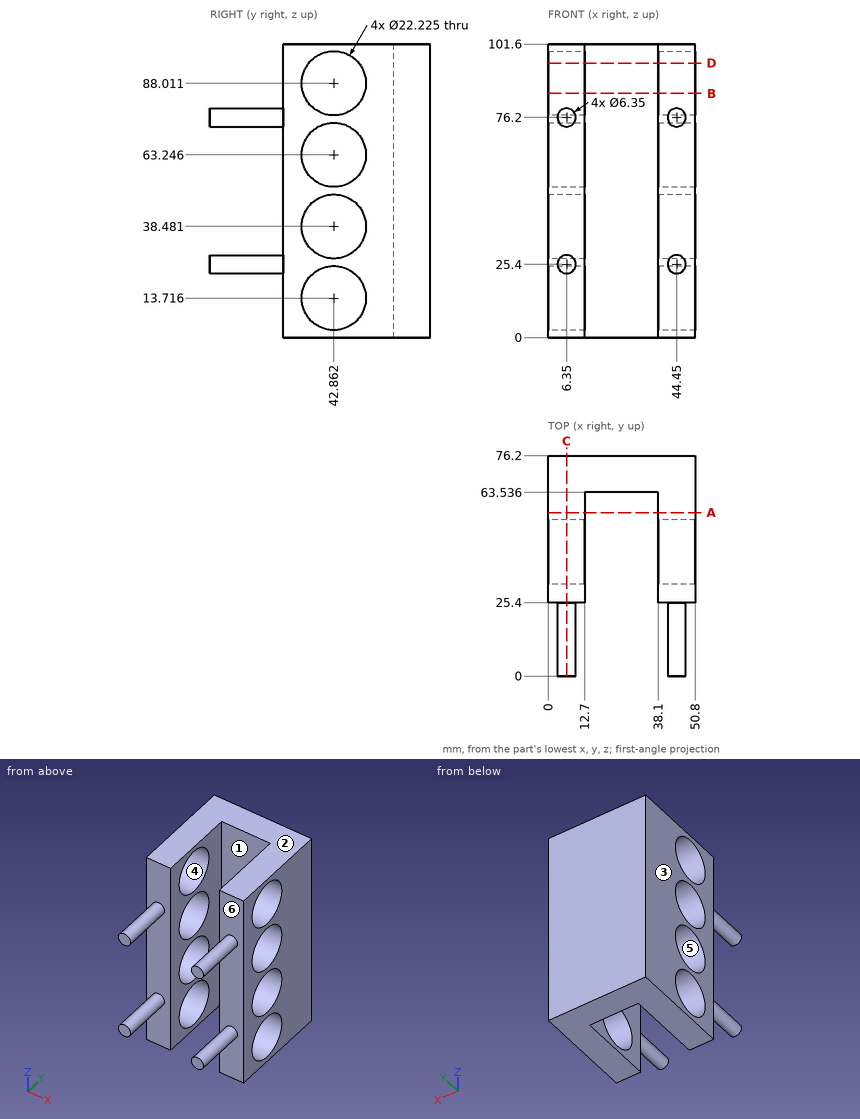
Geometry: see drawing. Coordinates: mm, zero at the bounding-box minimum. A direction names the side the tool comes from. Round coordinates to 2 decimals unless told otherwise and drop trailing zeros. Order: outer loops, then holes, each group sorted by start corner. A loop starts at its lowest first (then second) coordinate and runs counter-clockwise, first axis right, second up. Notation, with made-up numbers: (29, -2.75) -> (33, -2.75) arc R8 ccw to (33, 9.25) -> close; hole circle Ø5 at (-34, 89.25). An arc over 180 degrees is marked (long way). Answer as CSV lines item,"result".
Item 1: Section D-D, the plane z = 95. Return loops of the section in (x, y) (1 decimal).
A:
outline,"(0, 25.4) -> (12.7, 25.4) -> (12.7, 34.2) -> (0, 34.2) -> close; (0, 51.5) -> (12.7, 51.5) -> (12.7, 63.5) -> (38.1, 63.5) -> (38.1, 51.5) -> (50.8, 51.5) -> (50.8, 76.2) -> (0, 76.2) -> close; (38.1, 25.4) -> (50.8, 25.4) -> (50.8, 34.2) -> (38.1, 34.2) -> close"
Item 2: Reachability of the marked faces 1 and 2 from +Z, -Z, +X, -X, +Y, -Y: full face, straight path, thin tool, end or side. Return the list, or none.
A:
face 1,"+Z, -Z, -Y"
face 2,"+Z, +X, -X, +Y, -Y"
Item 3: Section B-B, the plane z = 84.5. Return loops of the section in (x, y) (1 decimal).
A:
outline,"(0, 25.4) -> (12.7, 25.4) -> (12.7, 32.3) -> (0, 32.3) -> close; (0, 53.4) -> (12.7, 53.4) -> (12.7, 63.5) -> (38.1, 63.5) -> (38.1, 53.4) -> (50.8, 53.4) -> (50.8, 76.2) -> (0, 76.2) -> close; (38.1, 25.4) -> (50.8, 25.4) -> (50.8, 32.3) -> (38.1, 32.3) -> close"
Item 4: Section C-C, the plane x = 6.35. Return loops of the section in (y, z) (1 decimal), plus the area to 3 significant figures.
A:
outline,"(0, 22.2) -> (25.4, 22.2) -> (25.4, 0) -> (76.2, 0) -> (76.2, 101.6) -> (25.4, 101.6) -> (25.4, 79.4) -> (0, 79.4) -> (0, 73) -> (25.4, 73) -> (25.4, 28.6) -> (0, 28.6) -> close; hole circle Ø22.2 at (42.9, 13.7); hole circle Ø22.2 at (42.9, 38.5); hole circle Ø22.2 at (42.9, 63.2); hole circle Ø22.2 at (42.9, 88)"
area,"3,930 mm²"
Item 5: Section A-A, the plane y = 56.5. Return loops of the section in (x, z), plus the area to 3 significant figures.
A:
outline,"(0, 0) -> (12.7, 0) -> (12.7, 101.6) -> (0, 101.6) -> close; (38.1, 0) -> (50.8, 0) -> (50.8, 101.6) -> (38.1, 101.6) -> close"
area,"2,580 mm²"
Item 6: Pin query (flat end, axial travel): pin 1 Ø10 at (x, z) = (19, 77.5) entering from -Y; pin 2 Ø6.5 at (x, z) = (46.5, 55) entering from -Y. Return the tip coordinate at first contact, or that it passes through.
A:
pin 1,"y = 63.54"
pin 2,"y = 25.4"
Item 7: Line query: L1, parallel to X at y = 28.5, z = 52; L2, parallel to X at y = 20.5, z = 76; L3, parallel to Y at x = 8, z = 50.5. Output: solid intervals per line, ascending.
A:
L1,"0 to 12.7, 38.1 to 50.8"
L2,"3.18 to 9.52, 41.28 to 47.62"
L3,"25.4 to 76.2"
Item 8: Pull-direction query (Y, two-part tool) for the marked faces 3, 4, 5 and 6; classes: pulls with the +Y half, pulls with the -Y half, needs draft (parallel to the pull), parting line crosses it, or undercut.
A:
face 3,"needs draft"
face 4,"undercut"
face 5,"undercut"
face 6,"pulls with the -Y half"
